Part model, mm, in its own coordinate system. A direction names the side the tool comes from. Give positions to 0.01 mm unless a question says otherwise; leave off trailing zeros. Order: outer loops, then holes, each group sorted by start corner. A loop starts at its lowest first (then second) coordinate and runs counter-clockwise, first axis right, second up. Notation, with made-up numbers: (-11, 17) - (43, 17) arc R11 cw to (43, 26) - close; hole circle Ø9 at (-8, 42.5). An arc over 180 degrees is marked (long way). One line per item, written item: value.
```python
from build123d import *

# Parameters (mm, degrees)
PAD_DEPTH       = 8
CHAMFER_SIZE    = 4
SKETCH001_R     = 1.7
POCKET_DEPTH    = 25.501
SKETCH002_R     = 3
POCKET001_DEPTH = 23.001


with BuildPart() as part:
    # Sketch → Pad (new body)
    with BuildSketch(Plane.XY):
        Polygon((0, 0), (23, 0), (23, 2.5), (2.5, 2.5), (2.5, 17.45), (25.5, 17.45), (25.5, 39.45), (2.5, 39.45), (2.5, 46.4), (0, 46.4), (0, 38.2), (3.2, 38.2), (3.2, 36.95), (23, 36.95), (23, 19.95), (3.2, 19.95), (3.2, 18.7), (0, 18.7), align=None)
    extrude(amount=PAD_DEPTH)

    # Chamfer
    chamfer_edges = [part.edges().sort_by_distance(p)[0] for p in [
        (2.5, 17.45, 4),
        (2.5, 39.45, 4),
        (2.5, 2.5, 4),
    ]]
    chamfer(chamfer_edges, length=CHAMFER_SIZE)

    # Sketch001 (on Face9 of Chamfer) → Pocket (cut, through all)
    with BuildSketch(Plane(origin=(0, 0, 0), x_dir=(0, -1, 0), z_dir=(-1, 0, 0))):
        with Locations((-42.7, 4)):
            Circle(SKETCH001_R)
        with Locations((-14.2, 4)):
            Circle(SKETCH001_R)
    extrude(amount=-POCKET_DEPTH, mode=Mode.SUBTRACT)

    # Sketch002 (on Face18 of Pocket) → Pocket001 (cut, through all)
    with BuildSketch(Plane.YZ.offset(2.5)):
        with Locations((14.2, 4)):
            Circle(SKETCH002_R)
        with Locations((42.7, 4)):
            Circle(SKETCH002_R)
    extrude(amount=POCKET001_DEPTH, mode=Mode.SUBTRACT)


solid = part.part
```
1) Which spindle directions (+Z, -Z, +X, -X, +Y, -Y) get a long thin tool onto all of the face, cutting with end or side? Do faces 1 (the face through (23, 29, 4)), 2 (the face through (4, 5, 4)), 3 (the face through (16, 39.45, 4)). Say none if no direction does.
Answer:
face 1: +Z, -Z, -X
face 2: +Z, -Z, +X
face 3: +Z, -Z, +X, +Y
2) Slice it at A-A on x = 14. Write the cut outline in (y, z).
Answer:
outline: (0, 0) - (2.5, 0) - (2.5, 8) - (0, 8) - close; (17.45, 0) - (19.95, 0) - (19.95, 8) - (17.45, 8) - close; (36.95, 0) - (39.45, 0) - (39.45, 8) - (36.95, 8) - close
3) Slice it at B-B on z = 4. Count the separate pieces of the cut face and the enclosed holes in it, then the cut area to 3 significant figures.
Answer:
separate pieces: 3
enclosed holes: 0
area: 267 mm2
4) Drop flat-ended pins along their axis: P1, Ø1, axis at x = 9.5, z = 6.5, coming from the +Y side; P2, Ø3, axis at y = 1, z = 4, coming from the +X side. Give the stop position or say it passes through.
Answer:
P1: stops at y = 39.45
P2: stops at x = 23
5) Slice it at C-C on y = 42.7. Write the cut outline in (x, z).
Answer:
outline: (0, 0) - (3.25, 0) - (3.25, 1) - (2.5, 1) - (2.5, 2.3) - (0, 2.3) - close; (0, 5.7) - (2.5, 5.7) - (2.5, 7) - (3.25, 7) - (3.25, 8) - (0, 8) - close
6) Wall check: line 1 along Y through (x, z) = (20, 3.5); line 2 along Z through (x, y) = (1.4, 42.7); line 3 along Y through (x, z) = (5, 4). Give the ranges that are in metal, low to high. Write a range as [from, to].
Answer:
line 1: y = [0, 2.5], [17.45, 19.95], [36.95, 39.45]
line 2: z = [0, 2.3], [5.7, 8]
line 3: y = [0, 4], [17.2, 19.95], [36.95, 39.7]
7) Two-plate mould, pull along Z, no slides. Class faces 4 (the face through (11, 0, 4)), 5 (the face through (12, 18, 8)), 6 (the face through (2.5, 11, 4)): pulls with the +Z half, pulls with the -Z half, needs draft (parallel to the pull), parting line crosses it, or undercut.
Answer:
face 4: needs draft
face 5: pulls with the +Z half
face 6: undercut
8) Slice it at D-D on y = 12. Write the cut outline in (x, z).
Answer:
outline: (0, 0) - (2.5, 0) - (2.5, 8) - (0, 8) - close
